Geometry: final body of the model. Coordinates: model frame, mm. Round coordinates to 2 decimals unless told otherwise and drop trailing zeros. Loops run counter-clockwise (first coordinate to the right, second up) from the corner with the lowest first, then second, coordinate; pieces in that order, holes last. Notation, with made-up numbers: (-20.5, -11) -> (5.5, -11) arc R25 ccw to (5.5, 15) -> close; hole circle Ø9 at (1, 74.25). An arc over 180 degrees is marked (long way). Answer in a Markdown table with one row per item.
Solid Edge part; units mm, degrees
sketch "Sketch1" plane through (0, 0, 0) normal (0, 0, 1) x (1, 0, 0)
  line L0 (-6.9282, -12) -> (6.9282, -12)
  line L1 (6.9282, -12) -> (13.8564, 0)
  line L2 (13.8564, 0) -> (6.9282, 12)
  line L3 (6.9282, 12) -> (-6.9282, 12)
  line L4 (-6.9282, 12) -> (-13.8564, 0)
  line L5 (-13.8564, 0) -> (-6.9282, -12)
extrude "Protrusion1" add sketch "Sketch1" along normal blind 7.5
sketch "Sketch2" plane through (0, 0, 0) normal (0, -1, 0) x (1, 0, 0)
  line L0 (-15.1213, 4.5223) -> (-10.8787, 8.7649)
  line L1 (-10.8787, 8.7649) -> (-19.9377, 8.7649)
  line L2 (-19.9377, 8.7649) -> (-19.9377, -1.2649)
  line L3 (-19.9377, -1.2649) -> (-10.8787, -1.2649)
  line L4 (-15.1213, 2.9777) -> (-10.8787, -1.2649)
  line L5 (-15.1213, 2.9777) -> (-15.1213, 4.5223)
revolve "RevolvedCutout1" cut sketch "Sketch2" angle 360 about axis through (0, 0, 57.15) along (0, 0, -1)
sketch "Sketch3" plane through (0, 0, 0) normal (0, 0, -1) x (1, 0, 0)
  circle A0 centre (0, 0) radius 7.5
extrude "Cutout1" cut sketch "Sketch3" against normal through all
properties part number "NutM15" material "Brass, yellow brass"
Item 1: Draft query along Y for faces 1 (the face through (5, 6, 7.5)), 2 (the face through (-7.493, -0.33, 3.698)), 3 (the face through (6.37, -10.91, 7.01)). Return one class per face: pulls with the +Y half, pulls with the -Y half, needs draft (parallel to the pull), parting line crosses it, or undercut.
Answer:
| item | result |
|---|---|
| face 1 | needs draft |
| face 2 | undercut |
| face 3 | pulls with the -Y half |
Item 2: Line query: probe 1 along Y at (x, z) = (0, 5.75); probe 2 along Y at (x, z) = (2.5, 7); probe 3 along X at (y, z) = (6.5, 5). Output: solid intervals per line, ascending. Write a range as [from, to].
Answer:
| item | result |
|---|---|
| probe 1 | y = [-12, -7.5], [7.5, 12] |
| probe 2 | y = [-12, -7.07], [7.07, 12] |
| probe 3 | x = [-10.1, -3.74], [3.74, 10.1] |
Item 3: Cut plane B-B (z = 3). Output: boundary loops of the cut face in (x, y), then the cut area to 3 significant figures.
Answer:
| item | result |
|---|---|
| outline | (-13.86, 0) -> (-6.93, -12) -> (6.93, -12) -> (13.86, 0) -> (6.93, 12) -> (-6.93, 12) -> close; hole circle Ø15 at (0, 0) |
| area | 322 mm² |
Item 4: Cut plane C-C (z = 1.25). Output: boundary loops of the cut face in (x, y).
Answer:
| item | result |
|---|---|
| outline | (-13.37, -0.85) -> (-7.42, -11.15) arc R13.39 ccw to (-5.95, -12) -> (5.95, -12) arc R13.39 ccw to (7.42, -11.15) -> (13.37, -0.85) arc R13.39 ccw to (13.37, 0.85) -> (7.42, 11.15) arc R13.39 ccw to (5.95, 12) -> (-5.95, 12) arc R13.39 ccw to (-7.42, 11.15) -> (-13.37, 0.85) arc R13.39 ccw to start; hole circle Ø15 at (0, 0) |
Item 5: Cut plane A-A (x = 0). Output: boundary loops of the cut face in (y, z).
Answer:
| item | result |
|---|---|
| outline | (-12, 0) -> (-7.5, 0) -> (-7.5, 7.5) -> (-12, 7.5) -> close; (7.5, 0) -> (12, 0) -> (12, 7.5) -> (7.5, 7.5) -> close |
Item 6: Pin query (flat end, axial travel): pin 1 Ø1.5 at (y, z) = (4.5, 1.5) entering from +X. Return the tip coordinate at first contact, or that it passes through.
Answer:
| item | result |
|---|---|
| pin 1 | stops at x = 11.69 |
